For this review, take the finished solid that the model builds, in its own axes (mm). Round coordinates to 2 decimals unless told otherwise and drop trailing zeros. Write each loop counter-clockwise with the first axis right and the second up, starting at its lowest first coordinate (ties: lowest second). Pieces come first, ordered by that corner, then holes.
from build123d import *

# Parameters (mm, degrees)
ESQUISSE1_R        = 3
ESQUISSE1_R_2      = 1.5
ESQUISSE1_R_3      = 6.25
ESQUISSE1_R_4      = 4
ESQUISSE1_R_5      = 11
BOSS_EXTRU_1_DEPTH = 5


with BuildPart() as part:
    # Esquisse1 → Boss.-Extru.1 (new body)
    with BuildSketch(Plane(origin=(0, 0, 0), x_dir=(1, 0, 0), z_dir=(0, 1, 0))):
        Polygon((-140, -95), (-140, 95), (-116, 130), (116, 130), (140, 95), (140, -95), (116, -130), (-116, -130), align=None)
        with Locations(Location((-130, 85, 0), (0, 0, 270))):
            Circle(ESQUISSE1_R, mode=Mode.SUBTRACT)
        with Locations(Location((-30, 10, 0), (0, 0, 270))):
            Circle(ESQUISSE1_R_2, mode=Mode.SUBTRACT)
        with Locations(Location((-50, 10, 0), (0, 0, 270))):
            Circle(ESQUISSE1_R_2, mode=Mode.SUBTRACT)
        with Locations(Location((-70, 10, 0), (0, 0, 270))):
            Circle(ESQUISSE1_R_2, mode=Mode.SUBTRACT)
        with Locations(Location((-90, 10, 0), (0, 0, 270))):
            Circle(ESQUISSE1_R_2, mode=Mode.SUBTRACT)
        with Locations(Location((-110, 10, 0), (0, 0, 270))):
            Circle(ESQUISSE1_R_2, mode=Mode.SUBTRACT)
        with Locations(Location((-130, 10, 0), (0, 0, 270))):
            Circle(ESQUISSE1_R_2, mode=Mode.SUBTRACT)
        with Locations(Location((-50, 30, 0), (0, 0, 270))):
            Circle(ESQUISSE1_R_2, mode=Mode.SUBTRACT)
        with Locations(Location((-70, 30, 0), (0, 0, 270))):
            Circle(ESQUISSE1_R_2, mode=Mode.SUBTRACT)
        with Locations(Location((-90, 30, 0), (0, 0, 270))):
            Circle(ESQUISSE1_R_2, mode=Mode.SUBTRACT)
        with Locations(Location((-110, 30, 0), (0, 0, 270))):
            Circle(ESQUISSE1_R_2, mode=Mode.SUBTRACT)
        with Locations(Location((-130, 30, 0), (0, 0, 270))):
            Circle(ESQUISSE1_R_2, mode=Mode.SUBTRACT)
        with Locations(Location((-100, -90, 0), (0, 0, 270))):
            Circle(ESQUISSE1_R_3, mode=Mode.SUBTRACT)
        with Locations(Location((100, -90, 0), (0, 0, 90))):
            Circle(ESQUISSE1_R_3, mode=Mode.SUBTRACT)
        with Locations(Location((-70, -90, 0), (0, 0, 270))):
            Circle(ESQUISSE1_R_4, mode=Mode.SUBTRACT)
        with Locations(Location((-110, 50, 0), (0, 0, 270))):
            Circle(ESQUISSE1_R_2, mode=Mode.SUBTRACT)
        with Locations(Location((-130, 50, 0), (0, 0, 270))):
            Circle(ESQUISSE1_R_2, mode=Mode.SUBTRACT)
        with Locations(Location((-30, -50, 0), (0, 0, 270))):
            Circle(ESQUISSE1_R_4, mode=Mode.SUBTRACT)
        with Locations(Location((70, -90, 0), (0, 0, 270))):
            Circle(ESQUISSE1_R_4, mode=Mode.SUBTRACT)
        with Locations(Location((-110, 70, 0), (0, 0, 270))):
            Circle(ESQUISSE1_R_2, mode=Mode.SUBTRACT)
        with Locations(Location((-130, 70, 0), (0, 0, 270))):
            Circle(ESQUISSE1_R_2, mode=Mode.SUBTRACT)
        with Locations(Location((-110, 90, 0), (0, 0, 270))):
            Circle(ESQUISSE1_R_2, mode=Mode.SUBTRACT)
        with Locations(Location((-30, 30, 0), (0, 0, 270))):
            Circle(ESQUISSE1_R_2, mode=Mode.SUBTRACT)
        with Locations(Location((-10, 30, 0), (0, 0, 270))):
            Circle(ESQUISSE1_R_2, mode=Mode.SUBTRACT)
        with Locations(Location((-10, 125, 0), (0, 0, 270))):
            Circle(ESQUISSE1_R_2, mode=Mode.SUBTRACT)
        with Locations(Location((-10, -70, 0), (0, 0, 90))):
            Circle(ESQUISSE1_R_2, mode=Mode.SUBTRACT)
        with Locations(Location((-10, -50, 0), (0, 0, 90))):
            Circle(ESQUISSE1_R_2, mode=Mode.SUBTRACT)
        with Locations(Location((-10, -30, 0), (0, 0, 90))):
            Circle(ESQUISSE1_R_2, mode=Mode.SUBTRACT)
        with Locations(Location((-30, -90, 0), (0, 0, 90))):
            Circle(ESQUISSE1_R_2, mode=Mode.SUBTRACT)
        with Locations(Location((-30, -70, 0), (0, 0, 90))):
            Circle(ESQUISSE1_R_2, mode=Mode.SUBTRACT)
        with Locations(Location((-30, -30, 0), (0, 0, 90))):
            Circle(ESQUISSE1_R_2, mode=Mode.SUBTRACT)
        with Locations(Location((-84.9, 125, 0), (0, 0, 270))):
            Circle(ESQUISSE1_R_2, mode=Mode.SUBTRACT)
        with Locations(Location((-60.8, 109.8, 0), (0, 0, 270))):
            Circle(ESQUISSE1_R_2, mode=Mode.SUBTRACT)
        with Locations(Location((-50, -90, 0), (0, 0, 90))):
            Circle(ESQUISSE1_R_2, mode=Mode.SUBTRACT)
        with Locations(Location((-130, -70, 0), (0, 0, 90))):
            Circle(ESQUISSE1_R_2, mode=Mode.SUBTRACT)
        with Locations(Location((-110, -70, 0), (0, 0, 90))):
            Circle(ESQUISSE1_R_2, mode=Mode.SUBTRACT)
        with Locations(Location((-90, -70, 0), (0, 0, 90))):
            Circle(ESQUISSE1_R_2, mode=Mode.SUBTRACT)
        with Locations(Location((-70, -70, 0), (0, 0, 90))):
            Circle(ESQUISSE1_R_2, mode=Mode.SUBTRACT)
        with Locations(Location((-50, -70, 0), (0, 0, 90))):
            Circle(ESQUISSE1_R_2, mode=Mode.SUBTRACT)
        with Locations(Location((-130, -50, 0), (0, 0, 90))):
            Circle(ESQUISSE1_R_2, mode=Mode.SUBTRACT)
        with Locations(Location((-110, -50, 0), (0, 0, 90))):
            Circle(ESQUISSE1_R_2, mode=Mode.SUBTRACT)
        with Locations(Location((-90, -50, 0), (0, 0, 90))):
            Circle(ESQUISSE1_R_2, mode=Mode.SUBTRACT)
        with Locations(Location((-70, -50, 0), (0, 0, 90))):
            Circle(ESQUISSE1_R_2, mode=Mode.SUBTRACT)
        with Locations(Location((-50, -50, 0), (0, 0, 90))):
            Circle(ESQUISSE1_R_2, mode=Mode.SUBTRACT)
        with Locations(Location((-130, -30, 0), (0, 0, 90))):
            Circle(ESQUISSE1_R_2, mode=Mode.SUBTRACT)
        with Locations(Location((-110, -30, 0), (0, 0, 90))):
            Circle(ESQUISSE1_R_2, mode=Mode.SUBTRACT)
        with Locations(Location((-90, -30, 0), (0, 0, 90))):
            Circle(ESQUISSE1_R_2, mode=Mode.SUBTRACT)
        with Locations(Location((-70, -30, 0), (0, 0, 90))):
            Circle(ESQUISSE1_R_2, mode=Mode.SUBTRACT)
        with Locations(Location((-50, -30, 0), (0, 0, 90))):
            Circle(ESQUISSE1_R_2, mode=Mode.SUBTRACT)
        with Locations(Location((-130, -10, 0), (0, 0, 90))):
            Circle(ESQUISSE1_R_2, mode=Mode.SUBTRACT)
        with Locations(Location((-110, -10, 0), (0, 0, 90))):
            Circle(ESQUISSE1_R_2, mode=Mode.SUBTRACT)
        with Locations(Location((-90, -10, 0), (0, 0, 90))):
            Circle(ESQUISSE1_R_2, mode=Mode.SUBTRACT)
        with Locations(Location((-70, -10, 0), (0, 0, 90))):
            Circle(ESQUISSE1_R_2, mode=Mode.SUBTRACT)
        with Locations(Location((-50, -10, 0), (0, 0, 90))):
            Circle(ESQUISSE1_R_2, mode=Mode.SUBTRACT)
        with Locations(Location((-30, -10, 0), (0, 0, 90))):
            Circle(ESQUISSE1_R_2, mode=Mode.SUBTRACT)
        with Locations(Location((-130, -85, 0), (0, 0, 90))):
            Circle(ESQUISSE1_R, mode=Mode.SUBTRACT)
        with Locations(Location((130, -85, 0), (0, 0, 270))):
            Circle(ESQUISSE1_R, mode=Mode.SUBTRACT)
        with Locations(Location((21, -88.5, 0), (0, 0, 270))):
            Circle(ESQUISSE1_R_2, mode=Mode.SUBTRACT)
        with Locations(Location((115, -88.5, 0), (0, 0, 270))):
            Circle(ESQUISSE1_R_2, mode=Mode.SUBTRACT)
        with Locations(Location((21, -53, 0), (0, 0, 270))):
            Circle(ESQUISSE1_R_2, mode=Mode.SUBTRACT)
        with Locations(Location((89, -53, 0), (0, 0, 270))):
            Circle(ESQUISSE1_R_2, mode=Mode.SUBTRACT)
        with Locations(Location((21, 18, 0), (0, 0, 270))):
            Circle(ESQUISSE1_R_2, mode=Mode.SUBTRACT)
        with Locations(Location((89, 18, 0), (0, 0, 270))):
            Circle(ESQUISSE1_R_2, mode=Mode.SUBTRACT)
        with Locations(Location((115, 18, 0), (0, 0, 270))):
            Circle(ESQUISSE1_R_2, mode=Mode.SUBTRACT)
        with Locations(Location((0, -90, 0), (0, 0, 270))):
            Circle(ESQUISSE1_R_5, mode=Mode.SUBTRACT)
        with Locations(Location((-60.8, 81.9, 0), (0, 0, 270))):
            Circle(ESQUISSE1_R_2, mode=Mode.SUBTRACT)
        with Locations(Location((-91.22, 76.78, 0), (0, 0, 270))):
            Circle(ESQUISSE1_R_2, mode=Mode.SUBTRACT)
        with Locations(Location((-8.7, 76.78, 0), (0, 0, 270))):
            Circle(ESQUISSE1_R_2, mode=Mode.SUBTRACT)
        with Locations(Location((130, -70, 0), (0, 0, 270))):
            Circle(ESQUISSE1_R_2, mode=Mode.SUBTRACT)
        with Locations(Location((50, -90, 0), (0, 0, 270))):
            Circle(ESQUISSE1_R_2, mode=Mode.SUBTRACT)
        with Locations(Location((30, -90, 0), (0, 0, 270))):
            Circle(ESQUISSE1_R_2, mode=Mode.SUBTRACT)
        with Locations(Location((10, -30, 0), (0, 0, 270))):
            Circle(ESQUISSE1_R_2, mode=Mode.SUBTRACT)
        with Locations(Location((10, -50, 0), (0, 0, 270))):
            Circle(ESQUISSE1_R_2, mode=Mode.SUBTRACT)
        with Locations(Location((10, -70, 0), (0, 0, 270))):
            Circle(ESQUISSE1_R_2, mode=Mode.SUBTRACT)
        with Locations(Location((10, 90, 0), (0, 0, 90))):
            Circle(ESQUISSE1_R_2, mode=Mode.SUBTRACT)
        with Locations(Location((10, 70, 0), (0, 0, 90))):
            Circle(ESQUISSE1_R_2, mode=Mode.SUBTRACT)
        with Locations(Location((10, 50, 0), (0, 0, 90))):
            Circle(ESQUISSE1_R_2, mode=Mode.SUBTRACT)
        with Locations(Location((10, 30, 0), (0, 0, 90))):
            Circle(ESQUISSE1_R_2, mode=Mode.SUBTRACT)
        with Locations(Location((30, 90, 0), (0, 0, 90))):
            Circle(ESQUISSE1_R_2, mode=Mode.SUBTRACT)
        with Locations(Location((110, 90, 0), (0, 0, 90))):
            Circle(ESQUISSE1_R_2, mode=Mode.SUBTRACT)
        with Locations(Location((90, 90, 0), (0, 0, 90))):
            Circle(ESQUISSE1_R_2, mode=Mode.SUBTRACT)
        with Locations(Location((70, 90, 0), (0, 0, 90))):
            Circle(ESQUISSE1_R_2, mode=Mode.SUBTRACT)
        with Locations(Location((50, 90, 0), (0, 0, 90))):
            Circle(ESQUISSE1_R_2, mode=Mode.SUBTRACT)
        with Locations(Location((130, 70, 0), (0, 0, 90))):
            Circle(ESQUISSE1_R_2, mode=Mode.SUBTRACT)
        with Locations(Location((130, 50, 0), (0, 0, 90))):
            Circle(ESQUISSE1_R_2, mode=Mode.SUBTRACT)
        with Locations(Location((130, 85, 0), (0, 0, 90))):
            Circle(ESQUISSE1_R, mode=Mode.SUBTRACT)
        with Locations(Location((0, 0, 0), (0, 0, 270))):
            Circle(ESQUISSE1_R, mode=Mode.SUBTRACT)
        with BuildLine():
            Line((135, 30), (135, -50))
            ThreePointArc((135, -50), (130, -55), (125, -50))
            Line((125, -50), (125, 30))
            ThreePointArc((125, 30), (130, 35), (135, 30))
        make_face(mode=Mode.SUBTRACT)
    extrude(amount=BOSS_EXTRU_1_DEPTH)


solid = part.part
(1) We need section B-B, the plane y = 2.5. State how many separate pieces and enclosed holes the cut face has, and give its area (3 significant figures).
Geometry check:
separate pieces: 1
enclosed holes: 88
area: 68,800 mm2
(2) Mouldability with a two-part tool opening along X and no side actions: class faces 1 (the face through (128.168, 2.465, 112.255)), 2 (the face through (-127.832, 2.465, 112.745)), 3 (the face through (-29, 0, -2)), 4 (the face through (0, 2, 79)) as pulls with the +X half, pulls with the -X half, needs draft (parallel to the pull), parting line crosses it, or undercut.
Geometry check:
face 1: pulls with the +X half
face 2: pulls with the -X half
face 3: needs draft
face 4: undercut
(3) We need section A-A, the plane z = 23. Give the boundary of the cut face in (x, y), and give its area (3 significant figures).
Geometry check:
outline: (-140, 0) - (125, 0) - (125, 5) - (-140, 5) - close; (135, 0) - (140, 0) - (140, 5) - (135, 5) - close
area: 1,350 mm2
(4) For line 1 along X through (y, z) = (1.45, 7); line 2 along X through (y, z) = (1.9, -70); line 3 along X through (y, z) = (4.3, -18), list the stretches that pass through material, from the lowest coordinate up.
Geometry check:
line 1: x = -140 to 125, 135 to 140
line 2: x = -140 to -131.5, -128.5 to -111.5, -108.5 to 8.5, 11.5 to 128.5, 131.5 to 140
line 3: x = -140 to 19.5, 22.5 to 87.5, 90.5 to 113.5, 116.5 to 125, 135 to 140
